Read the model definition and answer for the solid it produces. Units are mm, in the model's axes. Face numbers are marked on the shaded views. A direction names the side the tool comes from. Coordinates: 2 decimals unless noted, no trailing zeros. Loops run counter-clockwise (first coordinate to the right, second up) from the corner with the lowest first, then second, coordinate; pieces in that order, holes last.
from build123d import *

# Parameters (mm, degrees)
F0_R     = 172.5
F1_DEPTH = 29
F2_R     = 134.95
F3_DEPTH = 1.6
F4_R     = 11.2
F5_DEPTH = 30.601
F6_R     = 8.25
F7_DEPTH = 30.601


with BuildPart() as f1:
    # F0 (on Top) → F1 (new body)
    with BuildSketch(Plane.XY):
        Circle(F0_R)
    extrude(amount=F1_DEPTH)

    # F2 (on face) → F3 (join)
    with BuildSketch(Plane(origin=(0, 0, 0), x_dir=(1, 0, 0), z_dir=(0, 0, -1))):
        Circle(F2_R)
    extrude(amount=F3_DEPTH)

    # F4 (on face) → F5 (cut, through all)
    with BuildSketch(Plane.XY.offset(29)):
        with Locations((0, 149.25)):
            Circle(F4_R)
        with Locations((-105.535687, 105.535687)):
            Circle(F4_R)
        with Locations((-149.25, 0)):
            Circle(F4_R)
        with Locations((-105.535687, -105.535687)):
            Circle(F4_R)
        with Locations((0, -149.25)):
            Circle(F4_R)
        with Locations((105.535687, -105.535687)):
            Circle(F4_R)
        with Locations((149.25, 0)):
            Circle(F4_R)
        with Locations((105.535687, 105.535687)):
            Circle(F4_R)
    extrude(amount=-F5_DEPTH, mode=Mode.SUBTRACT)

    # F6 (on face) → F7 (cut, through all)
    with BuildSketch(Plane.XY.offset(29)):
        with Locations((-50, 0)):
            Circle(F6_R)
        with Locations((50, 0)):
            Circle(F6_R)
    extrude(amount=-F7_DEPTH, mode=Mode.SUBTRACT)


solid = f1.part
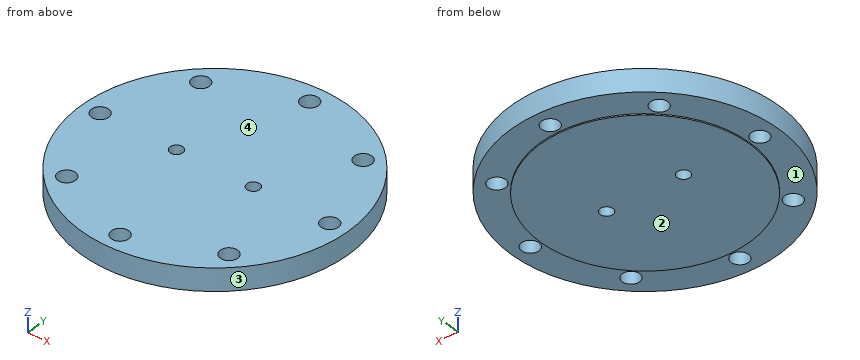
Q1. Straight lines are drawn through the part: probe 1 along Y at (x, z) = (-2.5, 21.5); probe 2 along Y at (x, z) = (-103, 1.5); probe 3 along Z at (x, y) = (124.5, -103). For each, find the intervals that lie inside material, in ascending order.
Findings below:
probe 1: y = -172.48 to -160.17, -138.33 to 138.33, 160.17 to 172.48
probe 2: y = -138.37 to -116.44, -94.63 to 94.63, 116.44 to 138.37
probe 3: z = 0 to 29
Q2. Flat-ended cylindrical pins translate along their axes: pin 1 Ø10 at (x, z) = (-71, 7.5) entering from -Y; pin 2 Ø1 at (x, z) = (-13.5, 12.5) entering from +Y; pin 3 Ø8 at (x, z) = (-58, 14.5) entering from +Y. Find the tip coordinate at first contact, or state that the pin passes through.
Findings below:
pin 1: stops at y = -159.37
pin 2: stops at y = 172.01
pin 3: stops at y = 163.83
Q3. A cutting plane is placed at B-B (y = 149.25). Give the vertices of the cut face in (x, z), then the cut area to 3 significant figures.
Findings below:
outline: (-86.49, 0) - (-11.2, 0) - (-11.2, 29) - (-86.49, 29) - close; (11.2, 0) - (86.49, 0) - (86.49, 29) - (11.2, 29) - close
area: 4,370 mm2
Q4. A cutting plane is placed at D-D (y = -123.5). Give the vertices of the cut face in (x, z).
Findings below:
outline: (-120.43, 0) - (-54.4, 0) - (-54.4, -1.6) - (54.4, -1.6) - (54.4, 0) - (120.43, 0) - (120.43, 29) - (-120.43, 29) - close
Q5. Determine the mould class of the marked faces 3 and 4 for opening direction Y: +Y half, -Y half, draft (parallel to the pull), parting line (faces both ways), or undercut.
Findings below:
face 3: parting line
face 4: draft
Q6. A cutting plane is placed at A-A (x = 0). Give the vertices of the cut face in (y, z), then the cut area to 3 significant figures.
Findings below:
outline: (-172.5, 0) - (-160.45, 0) - (-160.45, 29) - (-172.5, 29) - close; (-138.05, 0) - (-134.95, 0) - (-134.95, -1.6) - (134.95, -1.6) - (134.95, 0) - (138.05, 0) - (138.05, 29) - (-138.05, 29) - close; (160.45, 0) - (172.5, 0) - (172.5, 29) - (160.45, 29) - close
area: 9,140 mm2
Q7. Which of the six approach directions +Z, -Z, +X, -X, +Y, -Y give full straight-line access (tool end or side, diameter ignored) to the marked faces 1 and 2?
Findings below:
face 1: -Z
face 2: -Z, +X, -X, +Y, -Y
